Could you check a few things on this model? Use its own coordinates, in mm. A direction names the side the tool comes from. Coordinates: 2 decimals unless noted, no trailing zeros. Write each loop counter-clockwise with the first axis right and the second up, starting at its lowest first coordinate (ties: lowest second). Pieces come first, ordered by that corner, then holes.
Item 1: I want a section at C-C on x = 3. Please give me the cut outline in (y, z), then the cut area to 3 significant figures.
Item 2: I want a section at A-A on z = -3.25. Please give me the cut outline in (x, y).
Item 3: Thinking about a two-plate mould opening in Z: for faces 1 (the flat face through (-61, -2, 12.5)), 2 (the flat face through (12.75, -2, 0)), 3 (the flat face through (-63, -2, -12.5)), 4 (the flat face through (0, -2, 7.75)), which applies, +Z half, -Z half, draft (parallel to the pull), parting line (faces both ways), or undercut?
Item 4: I want a section at B-B on y = -2.1. Please give me the cut outline in (x, z), then the cut area to 3 significant figures.
Item 5: If I drill on probe 1 along X at (y, z) = (-1.4, -2.5); probe 2 along Z at (x, y) = (-119.5, -1.25), over which ranges is the centre line in solid material (lowest first)?
Item 6: Which directions (+Z, -Z, +X, -X, +Y, -Y) give clear straight access to the entire face, cutting with the end or side of a thin tool? Please do faces 5 (the flat face through (-132.25, -2, 0)), 6 (the flat face through (-63, -4, 0)).
from build123d import *

# Parameters (mm, degrees)
F0_W     = 15.5
F0_H     = 15.5
F1_DEPTH = 4


with BuildPart() as f1:
    # F0 (on Front) → F1 (new body)
    with BuildSketch(Plane.XZ):
        Polygon((12.75, -12.5), (12.75, 0), (12.75, 12.5), (-137.25, 12.5), (-137.25, -12.5), align=None)
        with Locations((-124.5, 0)):
            Rectangle(F0_W, F0_H, mode=Mode.SUBTRACT)
        Polygon((-7.75, 7.75), (7.75, 7.75), (7.75, 0), (7.75, -7.75), (-7.75, -7.75), align=None, mode=Mode.SUBTRACT)
    extrude(amount=F1_DEPTH)


solid = f1.part
Response values:
1. outline: (-4, -12.5) - (0, -12.5) - (0, -7.75) - (-4, -7.75) - close; (-4, 7.75) - (0, 7.75) - (0, 12.5) - (-4, 12.5) - close
1. area: 38.0 mm2
2. outline: (-137.25, -4) - (-132.25, -4) - (-132.25, 0) - (-137.25, 0) - close; (-116.75, -4) - (-7.75, -4) - (-7.75, 0) - (-116.75, 0) - close; (7.75, -4) - (12.75, -4) - (12.75, 0) - (7.75, 0) - close
3. face 1: +Z half
3. face 2: draft
3. face 3: -Z half
3. face 4: undercut
4. outline: (-137.25, -12.5) - (12.75, -12.5) - (12.75, 12.5) - (-137.25, 12.5) - close; hole (-132.25, -7.75) - (-116.75, -7.75) - (-116.75, 7.75) - (-132.25, 7.75) - close; hole (-7.75, -7.75) - (7.75, -7.75) - (7.75, 7.75) - (-7.75, 7.75) - close
4. area: 3,270 mm2
5. probe 1: x = -137.25 to -132.25, -116.75 to -7.75, 7.75 to 12.75
5. probe 2: z = -12.5 to -7.75, 7.75 to 12.5
6. face 5: +Y, -Y
6. face 6: +Z, -Z, +X, -X, -Y
